```python
from build123d import *

# Parameters (mm, degrees)
BOSS_EXTRUDE1_DEPTH = 107.95
BOSS_EXTRUDE2_DEPTH = 19.05
SKETCH1_4_R         = 63.5
SKETCH1_4_R_2       = 44.45
BOSS_EXTRUDE3_DEPTH = 127
SKETCH1_5_W         = 254
SKETCH1_5_H         = 50.8
BOSS_EXTRUDE4_DEPTH = 152.4


with BuildPart() as part:
    # Sketch1 → Boss-Extrude1 (new body)
    with BuildSketch(Plane.XY):
        with BuildLine():
            ThreePointArc((9.525, -62.781560788), (0, -63.5), (-9.525, -62.781560788))
            Line((-9.525, -62.781560788), (-9.525, -152.4))
            Line((-9.525, -152.4), (9.525, -152.4))
            Line((9.525, -152.4), (9.525, -62.781560788))
        make_face()
    extrude(amount=BOSS_EXTRUDE1_DEPTH)

    # Sketch1_3 → Boss-Extrude2 (add)
    with BuildSketch(Plane.XY):
        with BuildLine():
            ThreePointArc((-9.525, -62.781560788), (-48.15125907, -41.396935273), (-63.5, 0))
            Line((-63.5, 0), (-127, -152.4))
            Line((-127, -152.4), (-9.525, -152.4))
            Line((-9.525, -152.4), (-9.525, -62.781560788))
        make_face()
        with BuildLine():
            Line((127, -152.4), (63.5, 0))
            ThreePointArc((63.5, 0), (48.15125907, -41.396935273), (9.525, -62.781560788))
            Line((9.525, -62.781560788), (9.525, -152.4))
            Line((9.525, -152.4), (127, -152.4))
        make_face()
    extrude(amount=BOSS_EXTRUDE2_DEPTH)

    # Sketch1_4 → Boss-Extrude3 (add)
    with BuildSketch(Plane.XY):
        Circle(SKETCH1_4_R)
        Circle(SKETCH1_4_R_2, mode=Mode.SUBTRACT)
    extrude(amount=BOSS_EXTRUDE3_DEPTH)

    # Sketch1_5 → Boss-Extrude4 (add)
    with BuildSketch(Plane.XY):
        with Locations((0, -177.8)):
            Rectangle(SKETCH1_5_W, SKETCH1_5_H)
    extrude(amount=BOSS_EXTRUDE4_DEPTH)


solid = part.part
```
Input: part model. Units: mm. Frame: model coordinates. A direction names the side the tool comes from. Round coordinates to 2 decimals unless told otherwise and drop trailing zeros. Order: outer loops, then holes, each group sorted by start corner. A loop starts at its lowest first (then second) coordinate and runs counter-clockwise, first axis right, second up. Notation, with made-up numbers: (-25, 6) - (19, 6) arc R29 cw to (19, 34) - close; hole circle Ø7 at (57, 67.5). An arc over 180 degrees is marked (long way). Answer in a Markdown table with one row per item.
Item 1: Section query C-C (y = 13). Return the cut outline in (x, z), then the cut area to 3 significant figures.
Model answer:
| item | result |
|---|---|
| outline | (-62.16, 0) - (-42.51, 0) - (-42.51, 127) - (-62.16, 127) - close; (42.51, 0) - (62.16, 0) - (62.16, 127) - (42.51, 127) - close |
| area | 4,990 mm² |
Item 2: Line query: line 1 (Y direction, x = 0, z = 59); line 2 (Y direction, x = 38, z = 125); line 3 (Z direction, x = 56, y = -26.5). Output: solid intervals per line, ascending.
Model answer:
| item | result |
|---|---|
| line 1 | y = -203.2 to -44.45, 44.45 to 63.5 |
| line 2 | y = -203.2 to -152.4, -50.87 to -23.06, 23.06 to 50.87 |
| line 3 | z = 0 to 127 |
Item 3: Section query A-A (x = 0). Return the cut outline in (y, z), then the cut area to 3 significant figures.
Model answer:
| item | result |
|---|---|
| outline | (-203.2, 0) - (-44.45, 0) - (-44.45, 127) - (-63.5, 127) - (-63.5, 107.95) - (-152.4, 107.95) - (-152.4, 152.4) - (-203.2, 152.4) - close; (44.45, 0) - (63.5, 0) - (63.5, 127) - (44.45, 127) - close |
| area | 22,200 mm² |
Item 4: Section query D-D (x = -73). Return the cut outline in (y, z), then the cut area to 3 significant figures.
Model answer:
| item | result |
|---|---|
| outline | (-203.2, 0) - (-22.8, 0) - (-22.8, 19.05) - (-152.4, 19.05) - (-152.4, 152.4) - (-203.2, 152.4) - close |
| area | 10,200 mm² |
Item 5: Pin query (flat end, axial travel): pin 1 (12 mm diameter, centred on y = -129, z = 65.5, fed in from -X) (3 decimals); pin 2 (9.5 mm diameter, centred on x = -0.5, y = -105.5, fed in from +Z); pin 3 (6 mm diameter, centred on x = 36.5, z = 36.5, fed in from +Y). Return the tip coordinate at first contact, or that it passes through.
Model answer:
| item | result |
|---|---|
| pin 1 | stops at x = -9.525 |
| pin 2 | stops at z = 107.95 |
| pin 3 | stops at y = 53.94 |
Item 6: Section query B-B (z = 53). Return the cut outline in (x, y) (3 decimals), then the cut area to 3 significant figures.
Model answer:
| item | result |
|---|---|
| outline | (-127, -203.2) - (127, -203.2) - (127, -152.4) - (9.525, -152.4) - (9.525, -62.782) arc R63.5 ccw (long way) to (-9.525, -62.782) - (-9.525, -152.4) - (-127, -152.4) - close; hole circle Ø88.9 at (0, 0) |
| area | 21,100 mm² |
Item 7: Mould query, pull axis Y, two halves, no side actions, for faces 1 (the flat face through (-127, -178, 75)), 2 (the flat face through (95.694, -77.267, 9.392)), 3 (the flat face through (0, -107, 107.95)). Classes: released by +Y, released by -Y, zero draft, split by the parting line, or undercut.
Model answer:
| item | result |
|---|---|
| face 1 | zero draft |
| face 2 | released by +Y |
| face 3 | undercut |
Item 8: Reachability of faces 4 (the flat face through (-9.525, -107, 63)), 5 (the cylindrical face through (-8.27, 62.96, 62.61)), 6 (the flat face through (54, -92, 19.05)) from +Z, -Z, +X, -X, +Y, -Y: full face, straight path, thin tool, end or side. Return the list, or none.
Model answer:
| item | result |
|---|---|
| face 4 | +Z, -X |
| face 5 | +Z |
| face 6 | +Z, +X |
